Autodesk Inventor part; units mm, degrees
ref_plane "YZ Plane" through (0, 0, 0) normal (1, 0, 0) x (0, 1, 0)
ref_plane "XZ Plane" through (0, 0, 0) normal (0, 1, 0) x (-1, 0, 0)
ref_plane "XY Plane" through (0, 0, 0) normal (0, 0, 1) x (1, 0, 0)
sketch "Sketch1" plane through (0, 0, 0) normal (0, 1, 0) x (-1, 0, 0)
  line L0 (0, 0) -> (0, -61.8744)
  line L1 (0, 0) -> (-3.4036, 0)
  line L2 (0, -61.8744) -> (-3.4036, -61.8744)
  line L3 (-3.4036, 0) -> (-0.889, -15.5448)
  line L4 (-0.889, -15.5448) -> (-6.5786, -30.9015)
  line L5 (-6.5786, -30.9015) -> (-0.889, -46.3296)
  line L6 (-0.889, -46.3296) -> (-3.4036, -61.8744)
  dimension "d0" = 61.8744
  dimension "d1" = 3.4036
  dimension "d2" = 3.4036
  dimension "d3" = 15.5448
  dimension "d4" = 31.0642
  dimension "d5" = 15.5448
  dimension "d6" = 0.889
  dimension "d7" = 0.889
  dimension "d10" = 6.5786
extrude "Extrusion1" add sketch "Sketch1" along normal blind 7.3025
sketch "Sketch2" plane through (0, 0, 0) normal (0, 0, 1) x (1, 0, 0)
  line L0 (3.4036, 0) -> (0, 0)
  line L1 (1.651, 0) -> (0, 0)
  line L2 (0, 7.3025) -> (1.651, 7.3025)
  line L3 (1.651, 7.3025) -> (1.651, 0)
  line L4 (1.651, 0) -> (0, 0)
  line L5 (0, 0) -> (0, 7.3025)
  dimension "d17" = 1.651
sketch "Sketch3" plane through (3.4036, 0, -61.8744) normal (0, 0, -1) x (-1, 0, 0)
  line L0 (3.4036, 7.3025) -> (0, 7.3025)
  line L1 (0, 0) -> (3.4036, 0)
  line L2 (3.4036, 7.3025) -> (1.7526, 7.3025)
  line L3 (1.7526, 7.3025) -> (1.7526, 0)
  line L4 (1.7526, 0) -> (3.4036, 0)
  line L5 (3.4036, 0) -> (3.4036, 7.3025)
  dimension "d12" = 1.651
extrude "Extrusion2" add sketch "Sketch3" along normal blind 2.5654
extrude "Extrusion3" add sketch "Sketch2" along normal blind 2.5654
properties part number "short_insert_invert_CPY3"
Input: part model. Units: mm. Frame: model coordinates. A direction names the side the tool comes from. Round coordinates to 2 decimals unless told otherwise and drop trailing zeros. Write each loop counter-clockwise with the first axis right and the second up, starting at its lowest first coordinate (ties: lowest second). Pieces come first, ordered by that corner, then holes. Notation, with made-up numbers: (-27, 34) - (-15, 34) arc R18 cw to (-15, 43) - close; hole circle Ø9 at (-10, -33.5). An arc over 180 degrees is marked (long way). Write item = value, one per line.
(1) Pull-direction query (Z, two-part tool) for faces 1 (the flat face through (3, 4, -61.874)), 2 (the flat face through (1.651, 4, 1)), 3 (the flat face through (2.164, 3.6, -7.664)); classes: +Z half, -Z half, draft (parallel to the pull), parting line (faces both ways), or undercut.
Geometry check:
face_1 = -Z half
face_2 = draft
face_3 = undercut
(2) Section query D-D on x = 5.5. Output: boundary loops of the cut face in (y, z), then the cut area to 3 significant figures.
Geometry check:
outline = (0, -33.83) - (7.3, -33.83) - (7.3, -27.99) - (0, -27.99) - close
area = 42.6 mm^2
(3) Contact query for flat-ended pins moving along their axis: pin 1 Ø0.9 at (x, y) = (3, 2.5) entering from +Z; pin 2 Ø3 at (y, z) = (5, 1) entering from +X; pin 3 Ø1.5 at (y, z) = (5, -37) entering from +X. Output: stop coordinate, or through.
Geometry check:
pin_1 = 0
pin_2 = 3.4
pin_3 = 4.61
(4) Section query B-B on x = 2.25. Output: boundary loops of the cut face in (y, z), then the cut area to 3 significant figures.
Geometry check:
outline = (0, -61.87) - (7.3, -61.87) - (7.3, -54.74) - (0, -54.74) - close; (0, -42.64) - (7.3, -42.64) - (7.3, -19.22) - (0, -19.22) - close; (0, -7.13) - (7.3, -7.13) - (7.3, 0) - (0, 0) - close
area = 275 mm^2
(5) Access query for faces 4 (the flat face through (3, 4, 0)), 5 (the flat face through (1.651, 4, -63)), 6 (the flat face through (1, 4, 2.565)), 7 (the flat face through (1, 4, -64.44)), 8 (the flat face through (2.13, 3.6, -53.99)). Directions: +Z, -Z, +X, -X, +Y, -Y. A direction counts if a zero-diameter tool reaches every point of the face in a straight line with its end or side. Return the directions, or none.
Geometry check:
face_4 = +Z, +X, +Y, -Y
face_5 = -Z, +X, +Y, -Y
face_6 = +Z, +X, -X, +Y, -Y
face_7 = -Z, +X, -X, +Y, -Y
face_8 = +X, +Y, -Y
(6) Section query A-A on y = 1.25. Output: boundary loops of the cut face in (x, z), then the cut area to 3 significant figures.
Geometry check:
outline = (0, -64.44) - (1.65, -64.44) - (1.65, -61.87) - (3.4, -61.87) - (0.89, -46.33) - (6.58, -30.9) - (0.89, -15.54) - (3.4, 0) - (1.65, 0) - (1.65, 2.57) - (0, 2.57) - close
area = 190 mm^2
(7) Material intervals for probe 1 along X at (y, z) = (0.75, -55.5); probe 2 along X at (y, z) = (4.75, -35), sorted ascending.
Geometry check:
probe_1 = 0 to 2.37
probe_2 = 0 to 5.07
(8) Section query C-C on z = -33.5. Output: boundary loops of the cut face in (x, y), then the cut area to 3 significant figures.
Geometry check:
outline = (0, 0) - (5.62, 0) - (5.62, 7.3) - (0, 7.3) - close
area = 41.0 mm^2
